For this review, use the dimensioned drawing (mm, ordinates from the lowest corner) and the shaded views. Round coordinates to 2 decimals unless told otherwise and drop trailing zeros. Loops run counter-clockwise (first coordinate to the right, second up) from the corner with the lowest first, then second, coordinate; pieces in that order, holes last. Notation, with made-up numbers: (59.5, -33.75) - (71.5, -33.75) arc R31 ccw to (71.5, -6.75) - close; hole circle Ø10 at (58, 42). An arc over 180 degrees is marked (long way). Use one line per item in the form item = value. Start each with the question number.
(1) For pin 1 (0.9 mm diameter, centred on x = 22, z = 5, fed in from -Y), flat-tipped, find the tip position at first contact; note if it passes through.
(2) We need section A-A, the plane z = 7.75. Write out the cut boundary in (x, y).
(3) We need section B-B, the plane x = 22.5. Write out the cut boundary in (y, z).
(4) The part is to be moulded in two halves that separate along X. For the marked faces 1, 2 and 3, say which applies: released by +X, released by -X, zero draft, split by the parting line, or undercut.
(5) Wall thickness on probe 1 along X at (y, z) = (0.55, 0.5); probe 2 along X at (y, z) = (0.3, 0.75); probe 3 along Y at (x, z) = (22.75, 5): over which ranges is each line inside the solid? List them lowest first. Write a range as [from, to].
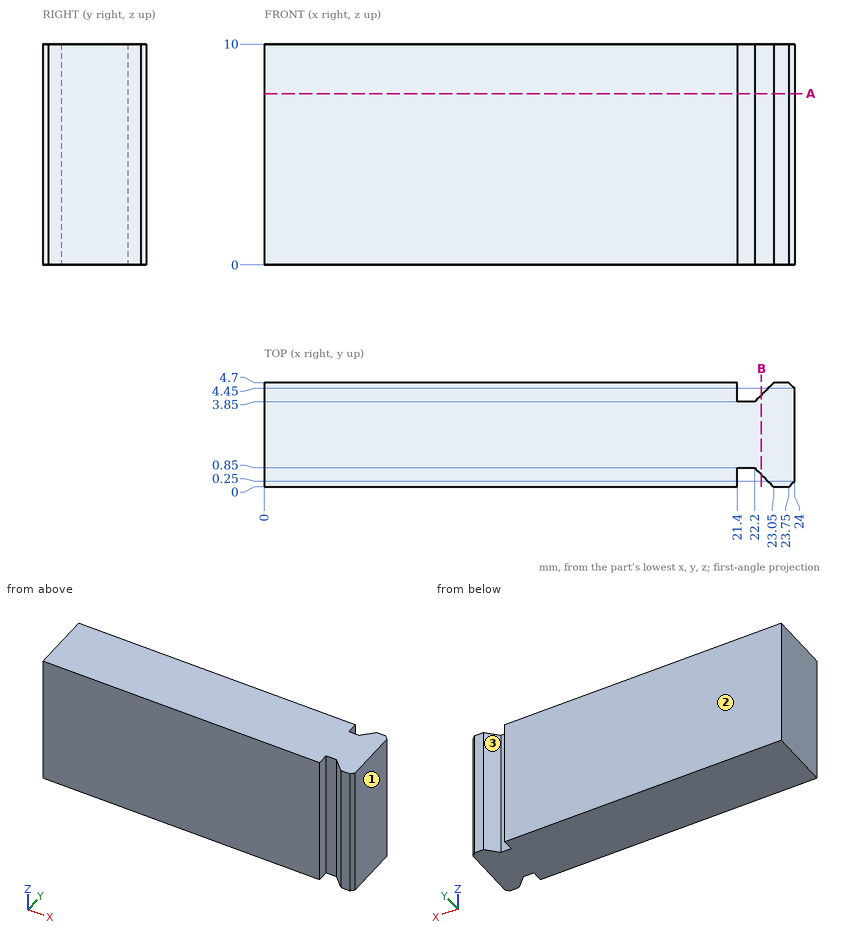
Data:
q1.pin_1 = 0.6
q2.outline = (0, 0) - (21.4, 0) - (21.4, 0.85) - (22.2, 0.85) - (23.05, 0) - (23.75, 0) - (24, 0.25) - (24, 4.45) - (23.75, 4.7) - (23.05, 4.7) - (22.2, 3.85) - (21.4, 3.85) - (21.4, 4.7) - (0, 4.7) - close
q3.outline = (0.55, 0) - (4.15, 0) - (4.15, 10) - (0.55, 10) - close
q4.face_1 = released by +X
q4.face_2 = zero draft
q4.face_3 = undercut
q5.probe_1 = [0, 21.4], [22.5, 24]
q5.probe_2 = [0, 21.4], [22.75, 24]
q5.probe_3 = [0.3, 4.4]
